from build123d import *

# Parameters (mm, degrees)
F0_W     = 100
F0_H     = 80
F1_DEPTH = 100
F2_T     = -5
F3_SIZE  = 2.5
F4_R     = 5


with BuildPart() as f1:
    # F0 (on Front) → F1 (new body)
    with BuildSketch(Plane.XZ):
        with Locations((1.5594035387, 1.0211700201)):
            Rectangle(F0_W, F0_H)
    extrude(amount=F1_DEPTH)

    # F2
    f2_openings = [f1.faces().sort_by_distance(p)[0] for p in [
        (1.559404, -50, 41.02117),
    ]]
    offset(amount=F2_T, openings=f2_openings)

    # F3
    f3_edges = [f1.edges().sort_by_distance(p)[0] for p in [
        (1.559404, -5, 41.02117),
        (-43.440596, -50, 41.02117),
        (1.559404, -95, 41.02117),
        (46.559404, -50, 41.02117),
    ]]
    chamfer(f3_edges, length=F3_SIZE)

    # F4
    f4_edges = [f1.edges().sort_by_distance(p)[0] for p in [
        (-48.440596, -100, 1.02117),
        (51.559404, -100, 1.02117),
        (51.559404, 0, 1.02117),
        (-48.440596, 0, 1.02117),
    ]]
    fillet(f4_edges, radius=F4_R)


solid = f1.part
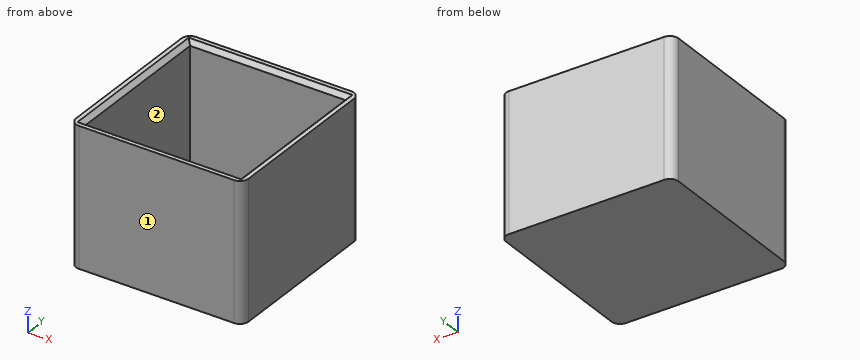
Could you check a few things on this model? Use its own coordinates, in mm. Face numbers are marked on the shaded views. A direction names the side the tool comes from. Give positions to 0.01 mm unless a question says otherwise; leave off trailing zeros. Order: outer loops, then holes, each group sorted by start corner. A loop starts at its lowest first (then second) coordinate and runs counter-clockwise, first axis right, second up.
1. For pin 1 (2 mm diameter, centred on x = 1, y = -85, fed in from +Z), with a flat end and sliding along its axis, tell me the tip position at first contact or that it passes through.
Answers below:
pin 1: stops at z = -33.98
2. Suppose I cut it at C-C (x = -25.5). Write out the boundary of the cut face in (y, z), plus the area to 3 significant figures.
Answers below:
outline: (-100, -38.98) - (0, -38.98) - (0, 41.02) - (-2.5, 41.02) - (-5, 38.52) - (-5, -33.98) - (-95, -33.98) - (-95, 38.52) - (-97.5, 41.02) - (-100, 41.02) - close
area: 1,240 mm2
3. I need wall thicknesses on L1, parallel to Y at x = 8.5, z = -9.5; L2, parallel to X at y = -19.5, z = 30; L3, parallel to Z at x = 5, y = -37.5. Which ranges of each line are inside material? Lowest first, please.
Answers below:
L1: y = -100 to -95, -5 to 0
L2: x = -48.44 to -43.44, 46.56 to 51.56
L3: z = -38.98 to -33.98
4. Suppose I cut it at B-B (y = -42). Write out the boundary of the cut face in (x, z), plus the area to 3 significant figures.
Answers below:
outline: (-48.44, -38.98) - (51.56, -38.98) - (51.56, 41.02) - (49.06, 41.02) - (46.56, 38.52) - (46.56, -33.98) - (-43.44, -33.98) - (-43.44, 38.52) - (-45.94, 41.02) - (-48.44, 41.02) - close
area: 1,240 mm2
5. Suppose I cut it at A-A (z = 3). Write out the boundary of the cut face in (x, y).
Answers below:
outline: (-48.44, -95) arc R5 ccw to (-43.44, -100) - (46.56, -100) arc R5 ccw to (51.56, -95) - (51.56, -5) arc R5 ccw to (46.56, 0) - (-43.44, 0) arc R5 ccw to (-48.44, -5) - close; hole (-43.44, -95) - (46.56, -95) - (46.56, -5) - (-43.44, -5) - close
6. Which directions (+Z, -Z, +X, -X, +Y, -Y) give clear straight access to the entire face, cutting with the end or side of a thin tool? Please do the marked faces 1 and 2.
Answers below:
face 1: +Z, -Z, +X, -X, -Y
face 2: +Z
